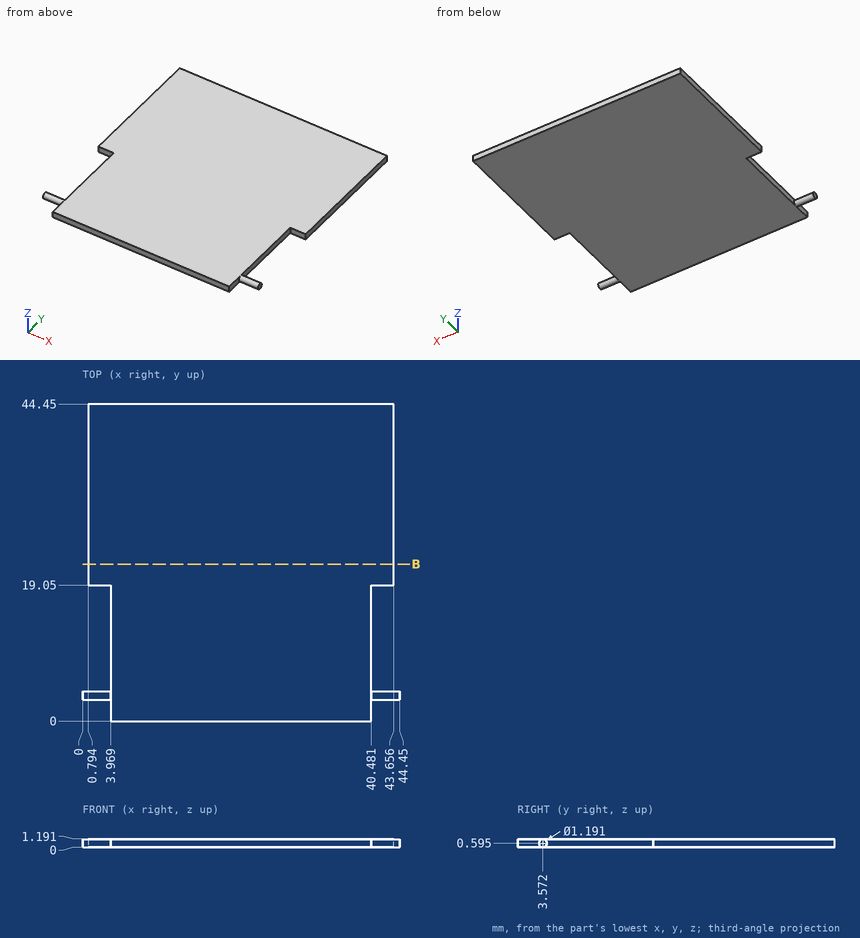
The figure shows three views and two pictorial views of one solid part (mm, origin at its lowest corner). Answer the questions. Coordinates: 2 decimals unless noted, no trailing zeros. Write each loop counter-clockwise with the first axis right and the second up, starting at its lowest first coordinate (ties: lowest second). Pieces come first, ordered by that corner, then holes. Notation, with made-up numbers: (-13, 69) -> (26, 69) arc R6 cw to (26, 79) -> close; hole circle Ø3 at (64.25, 54.25). An arc over 180 degrees is marked (long way). Return JSON: item names as keys, results as strings.
1. Find the intervals of material crossed by line 1 along X through (y, z) = (34, 0.95); line 2 along X through (y, z) = (19, 0.8), in increasing order. Write a range as from..to.
Found:
{"line 1": "0.79..43.66", "line 2": "3.97..40.48"}
2. Each of these flat-tipped pins is pushed along its axis until it touches: P1, Ø0.6, axis at y = 36.5, z = 0.5, coming from the -X side; P2, Ø0.6, axis at y = 11.5, z = 0.5, coming from the +X side; P3, Ø0.6, axis at y = 14, z = 0.5, coming from the -X side. Where does it stop, or does it pass through?
Found:
{"P1": "x = 0.79", "P2": "x = 40.48", "P3": "x = 3.97"}
3. A cutting plane is placed at B-B (y = 22). Determine the outline of the cut face in (x, z).
Found:
{"outline": "(0.79, 0) -> (43.66, 0) -> (43.66, 1.19) -> (0.79, 1.19) -> close"}
